Verification items for the finished model (mm, model axes). A direction names the side the tool comes from. Round coordinates to 2 decimals unless told otherwise and drop trailing zeros. Write each loop counter-clockwise with the first axis right and the second up, starting at its lowest first coordinate (ties: lowest second). Pieces come first, ordered by that corner, then holes. Notation, with made-up numbers: M 5.5,78.25 L 46.5,78.25 A20 ccw 46.5,112.25 Z; hole C 73,-10 d7. An arc over 180 degrees is marked long. One line per question, with ' | ' between items.
from build123d import *

# Parameters (mm, degrees)
SKETCH1_W           = 100
SKETCH1_H           = 150
BOSS_EXTRUDE1_DEPTH = 5
SKETCH2_W           = 100
SKETCH2_H           = 150
SKETCH2_W_2         = 90
SKETCH2_H_2         = 86
SKETCH2_H_3         = 50
BOSS_EXTRUDE2_DEPTH = 45


with BuildPart() as part:
    # Sketch1 → Boss-Extrude1 (new body)
    with BuildSketch(Plane.XY):
        Rectangle(SKETCH1_W, SKETCH1_H)
    extrude(amount=BOSS_EXTRUDE1_DEPTH)

    # Sketch2 → Boss-Extrude2 (add)
    with BuildSketch(Plane.XY.offset(5)):
        Rectangle(SKETCH2_W, SKETCH2_H)
        with Locations((0, 27)):
            Rectangle(SKETCH2_W_2, SKETCH2_H_2, mode=Mode.SUBTRACT)
        with Locations((0, -45)):
            Rectangle(SKETCH2_W_2, SKETCH2_H_3, mode=Mode.SUBTRACT)
    extrude(amount=BOSS_EXTRUDE2_DEPTH)


solid = part.part
1. Section check B-B, the plane y = 5. Record the cut outline in (x, z).
Results:
outline: M -50,0 L 50,0 L 50,50 L 45,50 L 45,5 L -45,5 L -45,50 L -50,50 Z
2. Section check C-C, the plane x = -17. Record the cut outline in (y, z).
Results:
outline: M -75,0 L 75,0 L 75,50 L 70,50 L 70,5 L -16,5 L -16,50 L -20,50 L -20,5 L -70,5 L -70,50 L -75,50 Z
3. Tool access check on faces 1 (the face through (-1, 70, 27)), 2 (the face through (-1, -75, 25)). Record the directions out of +Z, -Z, +X, -X, +Y, -Y that give a thin tool (end or side, any length) a straight path to the whole face; none if there is none.
Results:
face 1: +Z | face 2: +Z, -Z, +X, -X, -Y
4. Go/stop test with flat-tipped pins: P1, Ø1, axis at x = 8, y = 19.5, coming from the +Z side; P2, Ø12, axis at x = 7.5, y = -24, coming from the +Z side. Record where each tip stops, or that it passes through.
Results:
P1: stops at z = 5 | P2: stops at z = 50
5. Section check A-A, the plane z = 35.5. Record the cut outline in (x, y), then the cut area to 3 significant figures.
Results:
outline: M -50,-75 L 50,-75 L 50,75 L -50,75 Z; hole M -45,-70 L 45,-70 L 45,-20 L -45,-20 Z; hole M -45,-16 L 45,-16 L 45,70 L -45,70 Z | area: 2,760 mm2
6. Mould release check, pull along Y, two halves, no side actions. Record for faces 3 (the face through (45, 26, 27)), 4 (the face through (50, -1, 25)), 5 (the face through (-1, 75, 25)): pulls with the +Y half, pulls with the -Y half, needs draft (parallel to the pull), parting line crosses it, or undercut.
Results:
face 3: undercut | face 4: needs draft | face 5: pulls with the +Y half
7. Thickness scan on line 1 (Y direction, x = -32, z = 44); line 2 (X direction, y = -33, z = 31.5); line 3 (Z direction, x = -3, y = -0.5). Record the ranges inside material, lowest first.
Results:
line 1: y = -75 to -70, -20 to -16, 70 to 75 | line 2: x = -50 to -45, 45 to 50 | line 3: z = 0 to 5
